from build123d import *

# Parameters (mm, degrees)
BOX008_W     = 1
BOX008_H     = 8
BOX008_DEPTH = 9
BOX009_W     = 16
BOX009_H     = 1
BOX009_DEPTH = 9
BOX010_W     = 3
BOX010_H     = 1
BOX010_DEPTH = 3


with BuildPart() as box008:
    # Box008 → Box008 (new body)
    with BuildSketch(Plane(origin=(24, 1, 1), x_dir=(1, 0, 0), z_dir=(0, 0, 1))):
        with Locations((0.5, 4)):
            Rectangle(BOX008_W, BOX008_H)
    extrude(amount=BOX008_DEPTH)


with BuildPart() as box009:
    # Box009 → Box009 (new body)
    with BuildSketch(Plane(origin=(28, 8, 1), x_dir=(1, 0, 0), z_dir=(0, 0, 1))):
        with Locations((8, 0.5)):
            Rectangle(BOX009_W, BOX009_H)
    extrude(amount=BOX009_DEPTH)


with BuildPart() as fusion005:
    # Box010 → Box010 (new body)
    with BuildSketch(Plane(origin=(25, 8, 7), x_dir=(1, 0, 0), z_dir=(0, 0, 1))):
        with Locations((1.5, 0.5)):
            Rectangle(BOX010_W, BOX010_H)
    extrude(amount=BOX010_DEPTH)

    # Fusion005: union Box008, Box009
    add(box008.part)
    add(box009.part)


solid = fusion005.part
Check sheet for the modelled part. Datum: model origin and axes. Units: mm. A direction names the side the tool comes from. Give positions to 0.01 mm unless a question says otherwise; leave off trailing zeros. Write each loop counter-clockwise with the first axis right and the second up, starting at its lowest first coordinate (ties: lowest second). Pieces come first, ordered by that corner, then holes. Notation, with made-up numbers: (69, -30.75) -> (114, -30.75) arc R11 ccw to (114, -23.75) -> close; hole circle Ø4 at (7, -32). An arc over 180 degrees is marked (long way). One line per item, written item: value. Start each with the question number.
Item 1: Section check A-A on z = 4. Record the cut outline in (x, y), then the cut area to 3 significant figures.
Item 2: Gauge pin test, flat ends, axial feed: pin 1 (2.5 mm diameter, centred on x = 36.5, z = 3.5, fed in from -Y); pin 2 (2 mm diameter, centred on y = 4, z = 8.5, fed in from +X); pin 3 (0.8 mm diameter, centred on x = 27, y = 8.5, fed in from -Z). Record the tip position at first contact, or that the pin passes through.
Item 3: Material ranges on probe 1 along X at (y, z) = (6.75, 9.25); probe 2 along Y at (x, z) = (31, 2), recorded low to high. Write a range as from..to.
Item 4: Section check C-C on z = 8. Record the cut outline in (x, y), then the cut area to 3 significant figures.
Item 5: Section check B-B on y = 8.5. Record the cut outline in (x, z).
Item 6: Section check D-D on x = 27. Record the cut outline in (y, z).
Item 7: Tool access check on faces 1 (the flat face through (44, 8.5, 5.4)), 2 (the flat face through (26.5, 8.5, 7)). Record the directions out of +Z, -Z, +X, -X, +Y, -Y that give a thin tool (end or side, any length) a straight path to the whole face; none if there is none.
Item 8: Draft check along X on faces 3 (the flat face through (28, 8.5, 4)), 4 (the flat face through (34, 8, 5)), 5 (the flat face through (24, 5, 5)). Enter one of: +X half, -X half, draft (parallel to the pull), parting line (faces both ways), or undercut.
Results list:
1. outline: (24, 1) -> (25, 1) -> (25, 9) -> (24, 9) -> close; (28, 8) -> (44, 8) -> (44, 9) -> (28, 9) -> close
1. area: 24.0 mm²
2. pin 1: y = 8
2. pin 2: x = 25
2. pin 3: z = 7
3. probe 1: 24..25
3. probe 2: 8..9
4. outline: (24, 1) -> (25, 1) -> (25, 8) -> (44, 8) -> (44, 9) -> (24, 9) -> close
4. area: 27.0 mm²
5. outline: (24, 1) -> (25, 1) -> (25, 7) -> (28, 7) -> (28, 1) -> (44, 1) -> (44, 10) -> (24, 10) -> close
6. outline: (8, 7) -> (9, 7) -> (9, 10) -> (8, 10) -> close
7. face 1: +Z, -Z, +X, +Y, -Y
7. face 2: -Z, +Y, -Y
8. face 3: undercut
8. face 4: draft
8. face 5: -X half
